Work out the finished part from the listing and answer in its coordinate system (mm). A direction names the side the tool comes from. Coordinates: 2 decimals unless noted, no trailing zeros. Order: outer loops, then holes, each group sorted by start corner. A loop starts at its lowest first (then second) coordinate and runs counter-clockwise, first axis right, second up. Notation, with made-up numbers: (82, 13) - (126, 13) arc R18 ccw to (126, 30) - close; hole circle Ø6 at (-13, 84.5). An arc over 180 degrees is marked (long way). Use CSV: the item, a comma, the result in double quotes. Start each with the question number.
from build123d import *

# Parameters (mm, degrees)
SKETCH001_W    = 139
SKETCH001_H    = 87
PAD_DEPTH      = 25
THICKNESS_T    = 2
SKETCH002_R    = 5.947053
SKETCH002_R_2  = 6.391543
SKETCH002_R_3  = 7.479707
SKETCH002_R_4  = 6.690044
SKETCH002_R_5  = 7.551468
SKETCH002_R_6  = 6.341994
SKETCH002_R_7  = 8.509486
SKETCH002_R_8  = 9.409582
SKETCH002_R_9  = 8.069876
SKETCH002_R_10 = 7.030828
SKETCH002_R_11 = 5.146618
SKETCH002_R_12 = 6.982672
SKETCH002_R_13 = 7.752117
SKETCH002_R_14 = 10.787845
SKETCH002_R_15 = 5.65876
SKETCH002_R_16 = 3.93116
SKETCH002_R_17 = 3.377122
SKETCH002_R_18 = 5.622868
SKETCH002_R_19 = 3.905324
SKETCH002_R_20 = 4.228889
SKETCH002_R_21 = 3.528588
SKETCH002_R_22 = 3.16034
SKETCH002_R_23 = 6.106178
SKETCH002_R_24 = 4.85306
POCKET_DEPTH   = 5


with BuildPart() as part:
    # Sketch001 → Pad (new body)
    with BuildSketch(Plane.XY):
        with Locations((-29.136072, -13.994338)):
            Rectangle(SKETCH001_W, SKETCH001_H)
    extrude(amount=PAD_DEPTH)

    # Thickness
    thickness_openings = [part.faces().sort_by_distance(p)[0] for p in [
        (-98.636072, -13.994338, 12.5),
    ]]
    offset(amount=THICKNESS_T, openings=thickness_openings)

    # Sketch002 (on Face14 of Thickness) → Pocket (cut)
    with BuildSketch(Plane.XY.offset(27)):
        with Locations((-82.334571, 15.216334)):
            Circle(SKETCH002_R)
        with Locations((-61.021297, 18.021215)):
            Circle(SKETCH002_R_2)
        with Locations((-57.73288, -7.189993)):
            Circle(SKETCH002_R_3)
        with Locations((-86.232513, -9.656311)):
            Circle(SKETCH002_R_4)
        with Locations((-68.946266, -24.274019)):
            Circle(SKETCH002_R_5)
        with Locations((-82.723099, -44.663734)):
            Circle(SKETCH002_R_6)
        with Locations((-47.27071, -36.765015)):
            Circle(SKETCH002_R_7)
        with Locations((-30.922209, -11.599332)):
            Circle(SKETCH002_R_8)
        with Locations((-37.351395, 18.526012)):
            Circle(SKETCH002_R_9)
        with Locations((-17.329054, -28.866299)):
            Circle(SKETCH002_R_10)
        with Locations((-20.819183, -43.377895)):
            Circle(SKETCH002_R_11)
        with Locations((-12.920469, 15.403262)):
            Circle(SKETCH002_R_12)
        with Locations((9.489837, 16.872791)):
            Circle(SKETCH002_R_13)
        with Locations((-4.286991, -7.558129)):
            Circle(SKETCH002_R_14)
        with Locations((0, -29.968445)):
            Circle(SKETCH002_R_15)
        with Locations((-44.858665, 4.777251)):
            Circle(SKETCH002_R_16)
        with Locations((-74.249245, 5.328322)):
            Circle(SKETCH002_R_17)
        with Locations((-64.697304, -45.003048)):
            Circle(SKETCH002_R_18)
        with Locations((-36.225178, -46.839958)):
            Circle(SKETCH002_R_19)
        with Locations((-33.469814, -28.103462)):
            Circle(SKETCH002_R_20)
        with Locations((-49.450947, -18.551527)):
            Circle(SKETCH002_R_21)
        with Locations((-28.142773, 7.716309)):
            Circle(SKETCH002_R_22)
        with Locations((-5.732456, -45.003048)):
            Circle(SKETCH002_R_23)
        with Locations((-89.679298, -27.368698)):
            Circle(SKETCH002_R_24)
    extrude(amount=-POCKET_DEPTH, mode=Mode.SUBTRACT)


solid = part.part
1) The part is cut by section B-B on x = 4. Determine the outline of the cut face in (y, z), plus the area to 3 significant figures.
2) The part is cut by section A-A on z = 16. Determine the outline of the cut face in (x, y).
3) For faces 1 (the face through (-30, -13, 0)), 2 (the face through (42.364, -15, 12)), 3 (the face through (-54.925, 19.941, 26.014)), determine the directions among +Z, -Z, +X, -X, +Y, -Y from which every point of the face is accessible in a straight line to the end or side of a thin tool.
4) For a pull along X with two mould halves and no side action, classify faces 4 (the face through (-28.83, 4.63, 26.01)), 5 (the face through (-30, -23, 27)), 6 (the face through (40.364, -15, 12)) as +X half, -X half, draft (parallel to the pull), parting line (faces both ways), or undercut.
5) Straight lines are drawn through the part: line 1 (Z direction, x = -86, y = -17); line 2 (Y direction, x = -67, z = 0.25); line 3 (X direction, y = 20, z = 10.75). For each, find the intervals that lie inside material, in ascending order. Write a range as [from, to].
6) Flat-ended cylindrical pins translate along their axes: P1, Ø5.5, axis at x = -74.25, y = 5.33, coming from the +Z side; P2, Ø11, axis at x = -33.47, y = -28.1, coming from the +Z side; P3, Ø1, axis at y = 8.5, z = 18, coming from the -X side. Find the tip coordinate at first contact, or state that the pin passes through.
Answer key:
1,outline,"(-59.49, 0) arc R2 ccw to (-57.49, -2) - (29.51, -2) arc R2 ccw to (31.51, 0) - (31.51, 25) arc R2 ccw to (29.51, 27) - (22.35, 27) - (22.35, 25) - (29.51, 25) - (29.51, 0) - (-57.49, 0) - (-57.49, 25) - (-33.97, 25) - (-33.97, 27) - (-57.49, 27) arc R2 ccw to (-59.49, 25) - close; (-25.97, 25) - (-14.46, 25) - (-14.46, 27) - (-25.97, 27) - close; (-0.65, 25) - (11.4, 25) - (11.4, 27) - (-0.65, 27) - close"
1,area,"395 mm^2"
2,outline,"(-98.64, -59.49) - (40.36, -59.49) arc R2 ccw to (42.36, -57.49) - (42.36, 29.51) arc R2 ccw to (40.36, 31.51) - (-98.64, 31.51) - (-98.64, 29.51) - (40.36, 29.51) - (40.36, -57.49) - (-98.64, -57.49) - close"
3,face 1,"-X"
3,face 2,"+Z, -Z, +X, +Y, -Y"
3,face 3,"+Z"
4,face 4,"undercut"
4,face 5,"draft"
4,face 6,"-X half"
5,line 1,"[-2, 0], [25, 27]"
5,line 2,"[-59.49, -57.49], [29.51, 31.51]"
5,line 3,"[40.36, 42.36]"
6,P1,"z = 0"
6,P2,"z = 27"
6,P3,"x = 40.36"
